from build123d import *

# Parameters (mm, degrees)
SKETCH1_R           = 1.5
BOSS_EXTRUDE1_DEPTH = 1.6


with BuildPart() as part:
    # Sketch1 → Boss-Extrude1 (new body)
    with BuildSketch(Plane(origin=(0, 0, 0), x_dir=(1, 0, 0), z_dir=(0, 1, 0))):
        Polygon((-65, 52), (-27, 80), (0, 80), (0, -20), (-65, -20), align=None)
        with Locations((-43.840620434, 43.840620434)):
            Circle(SKETCH1_R, mode=Mode.SUBTRACT)
    boss_extrude1 = extrude(amount=BOSS_EXTRUDE1_DEPTH)

    # Mirror1: Boss-Extrude1 across plane
    add(boss_extrude1.mirror(Plane(origin=(0, 1.6, 20), x_dir=(0, 0, 1), z_dir=(-1, 0, 0))))


solid = part.part
Input: part model. Units: mm. Frame: model coordinates. Coordinates: 2 decimals unless noted, no trailing zeros. Loops run counter-clockwise (first coordinate to the right, second up) from the corner with the lowest first, then second, coordinate; pieces in that order, holes last. Notation, with made-up numbers: (8, 25) -> (36, 25) arc R11 cw to (36, 36) -> close; hole circle Ø6 at (20.25, 1.25). An arc over 180 degrees is marked (long way). One line per item, written item: value.
(1) Cut plane B-B (x = 35.5). Output: boundary loops of the cut face in (y, z), then the cut area to 3 significant figures.
Answer below:
outline: (0, -73.74) -> (1.6, -73.74) -> (1.6, 20) -> (0, 20) -> close
area: 150 mm2
(2) Cut plane A-A (y = 0.8). Output: boundary loops of the cut face in (x, z).
Answer below:
outline: (-65, -52) -> (-27, -80) -> (27, -80) -> (65, -52) -> (65, 20) -> (-65, 20) -> close; hole circle Ø3 at (-43.84, -43.84); hole circle Ø3 at (43.84, -43.84)
(3) Draft query along Z for faces 1 (the face through (-42.41, 0.79, -44.29)), 2 (the face through (-1, 0, -31)), 3 (the face through (42.41, 0.79, -44.29)), 4 (the face through (46, 1, -66)). Return one class per face: pulls with the +Z half, pulls with the -Z half, needs draft (parallel to the pull), parting line crosses it, or undercut.
Answer below:
face 1: undercut
face 2: needs draft
face 3: undercut
face 4: pulls with the -Z half
(4) Pin query (flat end, axial travel): pin 1 Ø3.5 at (x, z) = (-43.84, -43.84) entering from +Y. Return the tip coordinate at first contact, or that it passes through.
Answer below:
pin 1: stops at y = 1.6
(5) Ray query, line 1 along X through (y, z) = (0.5, -43); line 2 along Z through (x, y) = (49, 1.15); line 3 along X through (y, z) = (0.75, -62). Return the intervals inside material, ascending.
Answer below:
line 1: x = -65 to -45.08, -42.6 to 42.6, 45.08 to 65
line 2: z = -63.79 to 20
line 3: x = -51.43 to 51.43
